For this review, use the dimensioned drawing (mm, ordinates from the lowest corner) and the shaded views. A direction names the side the tool comes from. Round coordinates to 2 decimals unless told otherwise and drop trailing zeros. Loops run counter-clockwise (first coordinate to the right, second up) from the corner with the lowest first, then second, coordinate; pieces in that order, holes last. Notation, with made-up numbers: M 61.5,-38 L 67.5,-38 A29 cw 67.5,-7 Z; hole C -31,-21 d9. An arc over 180 degrees is marked long. Answer as a JSON object with one key per item and string values. Group by question number.
Item 1: Insertion check: P1, Ø2, axis at x = 5.5, z = 2.5, coming from the -Y side; P2, Ø8, axis at y = 42, z = 8.5, coming from the -X side; P3, Ø1.5, axis at x = 12.5, z = 8, coming from the +Y side. Each pin has a flat end and moves straight along its axis. Give the tip position at first contact, or say it passes through.
Item 2: Consider section C-C (z = 2). Give the boundary of the cut face in (x, y) (1 decimal).
Item 3: Consider section D-D (y = 23.5). Give the boundary of the cut face in (x, z), and give its area (3 significant figures).
Item 4: Consider section B-B (z = 10.5). Give the boundary of the cut face in (x, y) (1 decimal).
Item 5: To check wall thickness, follow line 1 (Z direction, x = 26, y = 8); line 2 (Y direction, x = 19, z = 2.5) (1 decimal); line 3 (Y direction, x = 23, z = 3.75) (1 decimal). State the ranges of each line that lie inside material, in increasing order.
Item 6: Consider section A-A (x = 15). Give the boundary of the cut face in (y, z) (1 decimal).
Item 7: Tool access review of the marked faces 1, 2, 3 and 4: name each direction out of +Z, -Z, +X, -X, +Y, -Y from which nothing blocks a thin tool from reaching the whole face with its end or side.
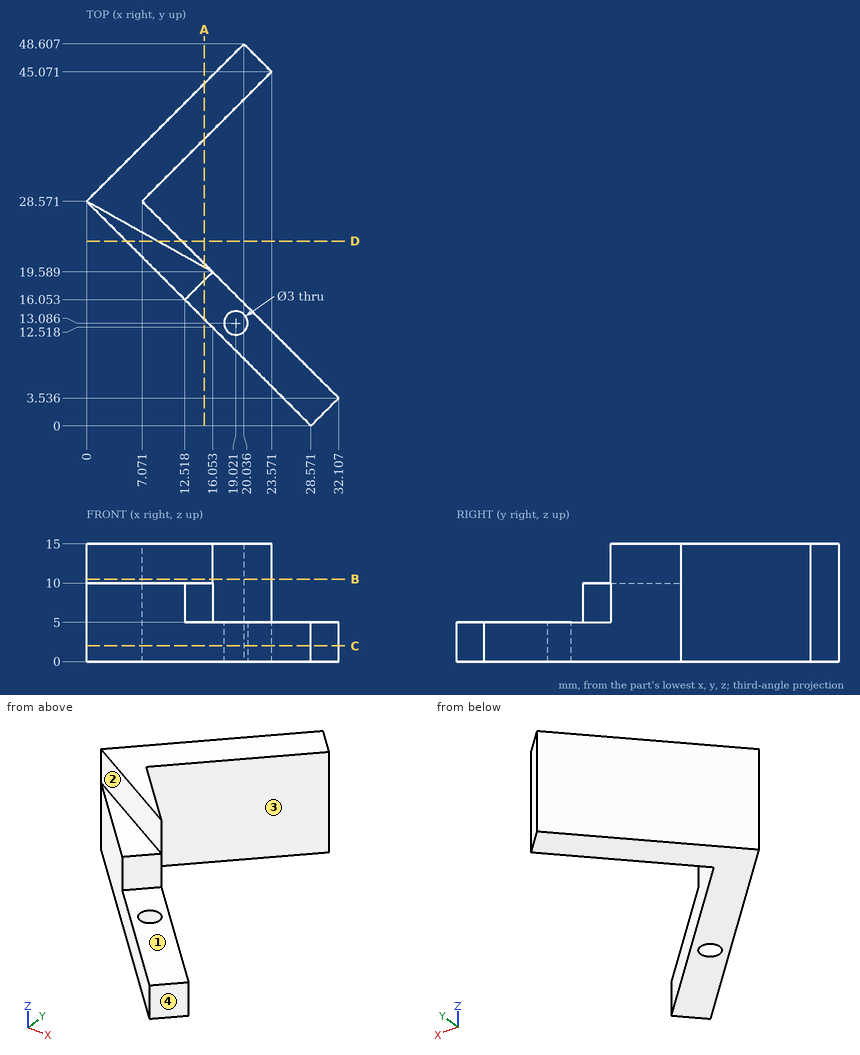
Geometry results:
{
 "1": {"P1": "stops at y = 22.07", "P2": "stops at x = 9.43", "P3": "stops at y = 41.82"},
 "2": {"outline": "M 0,28.6 L 28.6,0 L 32.1,3.5 L 7.1,28.6 L 23.6,45.1 L 20,48.6 Z; hole C 19,13.1 d3"},
 "3": {"outline": "M 5.07,0 L 12.14,0 L 12.14,15 L 9.06,15 L 9.06,10 L 5.07,10 Z", "area": "86.1 mm^2"},
 "4": {"outline": "M 0,28.6 L 16.1,19.6 L 7.1,28.6 L 23.6,45.1 L 20,48.6 Z"},
 "5": {"line 1": "z = 0 to 5", "line 2": "y = 9.6 to 11.6, 14.6 to 16.6, 40.5 to 47.6", "line 3": "y = 5.6 to 12.6, 44.5 to 45.6"},
 "6": {"outline": "M 13.6,0 L 20.6,0 L 20.6,15 L 20.2,15 L 20.2,10 L 18.5,10 L 18.5,5 L 13.6,5 Z; M 36.5,0 L 43.6,0 L 43.6,15 L 36.5,15 Z"},
 "7": {"face 1": "+Z, +X, -Y", "face 2": "+Z, -X, -Y", "face 3": "+Z, -Z, +X", "face 4": "+Z, -Z, +X, -Y"}
}
